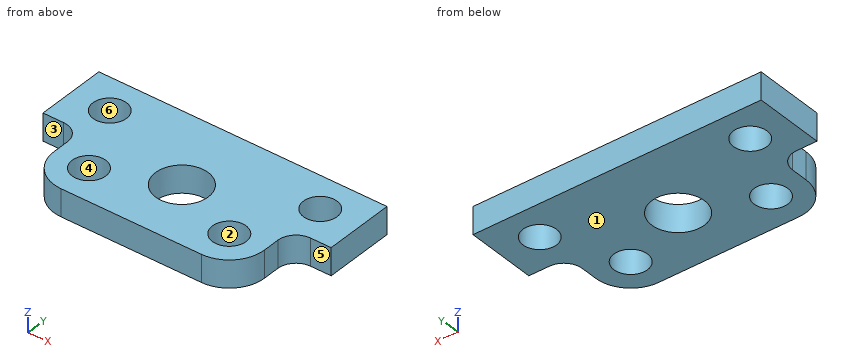
from build123d import *

# Parameters (mm, degrees)
F0_R     = 1.524
F0_R_2   = 2.38125
F0_R_3   = 1.519554
F1_DEPTH = 2.4638


with BuildPart() as f1:
    # F0 (on Top) → F1 (new body)
    with BuildSketch(Plane.XY):
        with BuildLine():
            ThreePointArc((-21.506696, 14.320038), (-20.57676, 12.074974), (-18.331696, 11.145038))
            Line((-18.331696, 11.145038), (-17.426178, 11.145038))
            Line((-17.426178, 11.145038), (-6.537213, 11.145038))
            Line((-6.537213, 11.145038), (-5.631696, 11.145038))
            ThreePointArc((-5.631696, 11.145038), (-3.386632, 12.074974), (-2.456696, 14.320038))
            Line((-2.456696, 14.320038), (-2.456696, 15.844038))
            ThreePointArc((-2.456696, 15.844038), (-1.973129, 17.011471), (-0.805696, 17.495038))
            Line((-0.805696, 17.495038), (-0.59268, 17.495038))
            Line((-0.59268, 17.495038), (1.05832, 17.495038))
            Line((1.05832, 17.495038), (1.05832, 19.146038))
            Line((1.05832, 19.146038), (1.05832, 22.194038))
            Line((1.05832, 22.194038), (1.05832, 23.845038))
            Line((1.05832, 23.845038), (-0.59268, 23.845038))
            Line((-0.59268, 23.845038), (-2.456696, 23.845038))
            Line((-2.456696, 23.845038), (-4.92218, 23.845038))
            Line((-4.92218, 23.845038), (-18.700644, 23.845038))
            Line((-18.700644, 23.845038), (-23.370711, 23.845038))
            Line((-23.370711, 23.845038), (-25.021711, 23.845038))
            Line((-25.021711, 23.845038), (-25.021711, 22.194038))
            Line((-25.021711, 22.194038), (-25.021711, 19.146038))
            Line((-25.021711, 19.146038), (-25.021711, 17.495038))
            Line((-25.021711, 17.495038), (-23.370711, 17.495038))
            Line((-23.370711, 17.495038), (-23.157696, 17.495038))
            ThreePointArc((-23.157696, 17.495038), (-21.990262, 17.011471), (-21.506696, 15.844038))
            Line((-21.506696, 15.844038), (-21.506696, 14.320038))
        make_face()
        with Locations((-18.331696, 14.320038)):
            Circle(F0_R, mode=Mode.SUBTRACT)
        with Locations((-5.631696, 14.320038)):
            Circle(F0_R, mode=Mode.SUBTRACT)
        with Locations((-11.936313, 16.847185)):
            Circle(F0_R_2, mode=Mode.SUBTRACT)
        with Locations((-21.506696, 20.670038)):
            Circle(F0_R_3, mode=Mode.SUBTRACT)
        with Locations((-2.456696, 20.670038)):
            Circle(F0_R_3, mode=Mode.SUBTRACT)
    extrude(amount=F1_DEPTH)


solid = f1.part
The listing builds one solid part. Answer for the finished solid, in the listing's coordinates (mm). Face numbers are marked on the shaded views. A direction names the side the tool comes from. Round coordinates to 2 decimals unless told otherwise and drop trailing zeros. Order: outer loops, then holes, each group sorted by start corner. A loop starts at its lowest first (then second) coordinate and runs counter-clockwise, first axis right, second up. Notation, with made-up numbers: (-37, -34.75) -> (-24, -34.75) arc R22 cw to (-24, 4.25) -> close; hole circle Ø5 at (-23.75, 87.25). An arc over 180 degrees is marked (long way). Put each result on its own line as item: value.
Q1. Consider line 1 along X through (y, z) = (15, 0.75); line 2 along X through (y, z) = (13, 0.1); line 3 along X through (y, z) = (15.5, 0.25). Determine where each line is inside the solid, lowest interval first.
Results list:
line 1: -21.51 to -19.7, -16.97 to -13.44, -10.43 to -7, -4.27 to -2.46
line 2: -21.22 to -19.09, -17.57 to -6.39, -4.87 to -2.74
line 3: -21.51 to -19.3, -17.37 to -13.9, -9.97 to -6.6, -4.67 to -2.46
Q2. Section D-D, the plane z = 1.95 is taken. Count the separate pieces of the cut face and the enclosed holes in it, and give its area (3 significant figures).
Results list:
separate pieces: 1
enclosed holes: 5
area: 237 mm^2
Q3. Which of the six approach directions +Z, -Z, +X, -X, +Y, -Y give full straight-line access (tool end or side, diameter ignored) to the marked faces 5 and 6?
Results list:
face 5: +Z, -Z, +X, -Y
face 6: +Z, -Z
Q4. Each of these flat-tipped pins is pushed along its axis until it touches: P1, Ø4.5, axis at x = -11.94, y = 16.85, coming from the -Z side; P2, Ø1.2, axis at y = 15, z = 1.5, coming from the +X side; P3, Ø0.9, axis at x = 0.5, z = 1.5, coming from the -Y side. Where does it stop, or does it pass through?
Results list:
P1: through
P2: x = -2.46
P3: y = 17.5
Q5. Determine the mould class of the marked faces 1, 2, 3 and 4 for opening direction Y: pulls with the +Y half, pulls with the -Y half, needs draft (parallel to the pull), parting line crosses it, or undercut.
Results list:
face 1: needs draft
face 2: undercut
face 3: pulls with the -Y half
face 4: undercut
Q6. Section B-B, the plane x = -12 is taken. Write down the section's boundary in (y, z), and give its area (3 significant figures).
Results list:
outline: (11.15, 0) -> (14.47, 0) -> (14.47, 2.46) -> (11.15, 2.46) -> close; (19.23, 0) -> (23.85, 0) -> (23.85, 2.46) -> (19.23, 2.46) -> close
area: 19.6 mm^2
Q7. Section C-C, the plane y = 21.5 is taken. Write down the section's boundary in (x, z), and give its area (3 significant figures).
Results list:
outline: (-25.02, 0) -> (-22.78, 0) -> (-22.78, 2.46) -> (-25.02, 2.46) -> close; (-20.23, 0) -> (-3.73, 0) -> (-3.73, 2.46) -> (-20.23, 2.46) -> close; (-1.18, 0) -> (1.06, 0) -> (1.06, 2.46) -> (-1.18, 2.46) -> close
area: 51.7 mm^2
Q8. Section A-A, the plane y = 15.5 is taken. Write down the section's boundary in (x, z), and give its area (3 significant figures).
Results list:
outline: (-21.51, 0) -> (-19.3, 0) -> (-19.3, 2.46) -> (-21.51, 2.46) -> close; (-17.37, 0) -> (-13.9, 0) -> (-13.9, 2.46) -> (-17.37, 2.46) -> close; (-9.97, 0) -> (-6.6, 0) -> (-6.6, 2.46) -> (-9.97, 2.46) -> close; (-4.67, 0) -> (-2.46, 0) -> (-2.46, 2.46) -> (-4.67, 2.46) -> close
area: 27.8 mm^2
